Source: CAD feature listing. Evaluate the final solid. Frame: model axes, mm. Give positions to 0.01 mm unless a question says otherwise; leave off trailing zeros. Order: outer loops, then holes, each group sorted by start corner. A loop starts at its lowest first (then second) coordinate and runs counter-clockwise, first axis right, second up. Notation, with made-up numbers: (15.25, 37) - (36.25, 37) arc R30 ccw to (36.25, 69) - close; hole circle Ø8 at (65, 85.5). An arc over 180 degrees is marked (long way). Use CSV: the item, a comma, the result in double quotes.
```python
from build123d import *

# Parameters (mm, degrees)
F0_W     = 263
F0_H     = 480
F1_DEPTH = 22
F2_SIZE  = 21.99999


# Not quite as in the source:
# - a fillet or chamfer is up to 0.001 mm smaller than in the source, because OpenCascade refuses the exact size


with BuildPart() as f1:
    # F0 (on Right) → F1 (new body)
    with BuildSketch(Plane.YZ):
        Rectangle(F0_W, F0_H)
    extrude(amount=F1_DEPTH)

    # F2 (size 22 in the source; OpenCascade refuses exactly that, so slightly less here)
    f2_edges = [f1.edges().sort_by_distance(p)[0] for p in [
        (22, -131.5, 0),
        (22, 0, -240),
        (22, 131.5, 0),
        (22, 0, 240),
    ]]
    chamfer(f2_edges, length=F2_SIZE)


solid = f1.part
```
Item 1: Section C-C on x = 13.75. Return the cut outline in (y, z), then the cut area to 3 significant figures.
Filled in:
outline,"(-117.75, -226.25) - (117.75, -226.25) - (117.75, 226.25) - (-117.75, 226.25) - close"
area,"107,000 mm2"
Item 2: First-contact query: pin 1 (12 mm diameter, centred on x = 14.5, z = 104.5, fed in from +Y); pin 2 (12 mm diameter, centred on x = 10, z = 90, fed in from -Y); pin 3 (3 mm diameter, centred on x = 6.5, z = 179.5, fed in from +Y). Flat tips, straight axial feed; report the tip coordinate or a pass-through.
Filled in:
pin 1,"stops at y = 123"
pin 2,"stops at y = -127.5"
pin 3,"stops at y = 126.5"
Item 3: Material intervals for line 1 (Y direction, x = 2.5, z = -146); line 2 (Y direction, x = 18.75, z = -153.5); line 3 (Z direction, x = 19, y = 36.5), sorted ascending. Write a range as from..to.
Filled in:
line 1,"y = -129..129"
line 2,"y = -112.75..112.75"
line 3,"z = -221..221"
